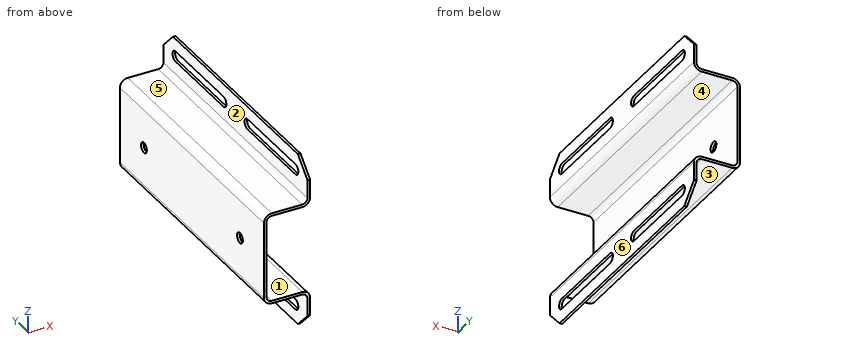
from build123d import *

# Parameters (mm, degrees)
BASE_FLANGE1_DEPTH = 150
CHAMFER1_SIZE      = 10
SKETCH6_R          = 3
CUT_EXTRUDE1_DEPTH = 10
CUT_EXTRUDE2_DEPTH = 10


# Sheet-metal steps are written as plain solids
with BuildPart() as part:
    # Sketch1 → Base-Flange1 (new body)
    with BuildSketch(Plane(origin=(0, 0, 0), x_dir=(1, 0, 0), z_dir=(0, 1, 0))):
        with BuildLine():
            Line((25, -25), (25, -4.5))
            ThreePointArc((25, -4.5), (23.681980515, -1.318019485), (20.5, 0))
            Line((20.5, 0), (3, 0))
            ThreePointArc((3, 0), (0.878679656, 0.878679656), (0, 3))
            Line((0, 3), (0, 47))
            ThreePointArc((0, 47), (0.878679656, 49.121320344), (3, 50))
            Line((3, 50), (20.5, 50))
            ThreePointArc((20.5, 50), (23.681980515, 51.318019485), (25, 54.5))
            Line((25, 54.5), (25, 75))
            Line((25, 75), (23.5, 75))
            Line((23.5, 75), (23.5, 54.5))
            ThreePointArc((23.5, 54.5), (22.621320344, 52.378679656), (20.5, 51.5))
            Line((20.5, 51.5), (3, 51.5))
            ThreePointArc((3, 51.5), (-0.181980515, 50.181980515), (-1.5, 47))
            Line((-1.5, 47), (-1.5, 3))
            ThreePointArc((-1.5, 3), (-0.181980515, -0.181980515), (3, -1.5))
            Line((3, -1.5), (20.5, -1.5))
            ThreePointArc((20.5, -1.5), (22.621320344, -2.378679656), (23.5, -4.5))
            Line((23.5, -4.5), (23.5, -25))
            Line((23.5, -25), (25, -25))
        make_face()
    extrude(amount=BASE_FLANGE1_DEPTH)

    # Chamfer1
    chamfer1_edges = [part.edges().sort_by_distance(p)[0] for p in [
        (24.25, 0, -75),
        (24.25, 0, 25),
        (24.25, 150, -75),
        (24.25, 150, 25),
    ]]
    chamfer(chamfer1_edges, length=CHAMFER1_SIZE)

    # Sketch6 → Cut-Extrude1 (cut)
    with BuildSketch(Plane.ZY.offset(1.5)):
        with Locations((-25, 25)):
            Circle(SKETCH6_R)
        with Locations((-25, 125)):
            Circle(SKETCH6_R)
    extrude(amount=-CUT_EXTRUDE1_DEPTH, mode=Mode.SUBTRACT)

    # Sketch7 → Cut-Extrude2 (cut)
    with BuildSketch(Plane.ZY.offset(-23.5)):
        with BuildLine():
            Line((-67.75, 12.5), (-67.75, 62.5))
            ThreePointArc((-67.75, 62.5), (-64.75, 65.5), (-61.75, 62.5))
            Line((-61.75, 62.5), (-61.75, 12.5))
            ThreePointArc((-61.75, 12.5), (-64.75, 9.5), (-67.75, 12.5))
        make_face()
        with BuildLine():
            Line((-67.75, 137.5), (-67.75, 87.5))
            ThreePointArc((-67.75, 87.5), (-64.75, 84.5), (-61.75, 87.5))
            Line((-61.75, 87.5), (-61.75, 137.5))
            ThreePointArc((-61.75, 137.5), (-64.75, 140.5), (-67.75, 137.5))
        make_face()
        with BuildLine():
            Line((17.75, 137.5), (17.75, 87.5))
            ThreePointArc((17.75, 87.5), (14.75, 84.5), (11.75, 87.5))
            Line((11.75, 87.5), (11.75, 137.5))
            ThreePointArc((11.75, 137.5), (14.75, 140.5), (17.75, 137.5))
        make_face()
        with BuildLine():
            Line((17.75, 12.5), (17.75, 62.5))
            ThreePointArc((17.75, 62.5), (14.75, 65.5), (11.75, 62.5))
            Line((11.75, 62.5), (11.75, 12.5))
            ThreePointArc((11.75, 12.5), (14.75, 9.5), (17.75, 12.5))
        make_face()
    extrude(amount=-CUT_EXTRUDE2_DEPTH, mode=Mode.SUBTRACT)


solid = part.part
Source: CAD feature listing. Evaluate the final solid. Frame: model axes, mm. Face numbers are marked on the shaded views. A direction names the side the tool comes from. Coordinates: 2 decimals unless noted, no trailing zeros. Order: outer loops, then holes, each group sorted by start corner. A loop starts at its lowest first (then second) coordinate and runs counter-clockwise, first axis right, second up. Notation, with made-up numbers: M -9,-37.5 L 22,-37.5 A16 cw 22,-27.5 Z; hole C -31.75,45.25 d7. An arc over 180 degrees is marked long. Write each question's results on one line, items separated by ' | '. Start each with the question number.
Item 1: Cut plane C-C (z = -25). Return loops of the section in (x, y).
Item 2: Cut plane A-A (y = 98.5). Return loops of the section in (x, z), and give its area (3 significant figures).
Item 3: First-contact query: pin 1 Ø8 at (y, z) = (32.5, -2.5) entering from +X; pin 2 Ø8 at (x, y) = (7, 26) entering from +Z; pin 3 Ø6 at (y, z) = (47.5, 2) entering from -X. Flat tips, straight axial feed; report the tip coordinate or a pass-through.
Item 4: Cut plane D-D (y = 125). Count the separate pieces of the cut face and the enclosed holes in it, and give its area (3 significant figures).
Item 5: Set-up query: the marked faces 4, 5 and 6. Return all of +Z, -Z, +X, -X, +Y, -Y with unobstructed straight access to the full face (end or side cutting, diameter ignored); none if empty.
Item 6: Cut plane B-B (x = 6.5). Return loops of the section in (y, z), and give its area (3 significant figures).
Item 7: Line query: probe 1 along Y at (x, z) = (-0.65, -25); probe 2 along Z at (x, y) = (7.25, 79.5); probe 3 along Z at (x, y) = (2, 40). Output: solid intervals per line, ascending.
Item 8: Draft query along Z for the marked faces 1, 2 and 3. Return one class per face: pulls with the +Z half, pulls with the -Z half, needs draft (parallel to the pull), parting line crosses it, or undercut.
Checked values:
1) outline: M -1.5,0 L 0,0 L 0,22 L -1.5,22 Z; M -1.5,28 L 0,28 L 0,122 L -1.5,122 Z; M -1.5,128 L 0,128 L 0,150 L -1.5,150 Z
2) outline: M -1.5,-47 A4.5 ccw 3,-51.5 L 20.5,-51.5 A3 cw 23.5,-54.5 L 23.5,-61.75 L 25,-61.75 L 25,-54.5 A4.5 ccw 20.5,-50 L 3,-50 A3 cw 0,-47 L 0,-3 A3 cw 3,0 L 20.5,0 A4.5 ccw 25,4.5 L 25,11.75 L 23.5,11.75 L 23.5,4.5 A3 cw 20.5,1.5 L 3,1.5 A4.5 ccw -1.5,-3 Z; M 23.5,-75 L 25,-75 L 25,-67.75 L 23.5,-67.75 Z; M 23.5,17.75 L 25,17.75 L 25,25 L 23.5,25 Z | area: 197 mm2
3) pin 1: stops at x = 23.85 | pin 2: stops at z = 1.5 | pin 3: stops at x = -1.03
4) separate pieces: 4 | enclosed holes: 0 | area: 188 mm2
5) face 4: +X, +Y, -Y | face 5: +Z, -X, +Y, -Y | face 6: +Z, -Z, +X, +Y, -Y
6) outline: M 0,-51.5 L 150,-51.5 L 150,-50 L 0,-50 Z; M 0,0 L 150,0 L 150,1.5 L 0,1.5 Z | area: 450 mm2
7) probe 1: y = 0 to 22, 28 to 122, 128 to 150 | probe 2: z = -51.5 to -50, 0 to 1.5 | probe 3: z = -51.39 to -49.83, -0.17 to 1.39
8) face 1: undercut | face 2: needs draft | face 3: pulls with the -Z half
